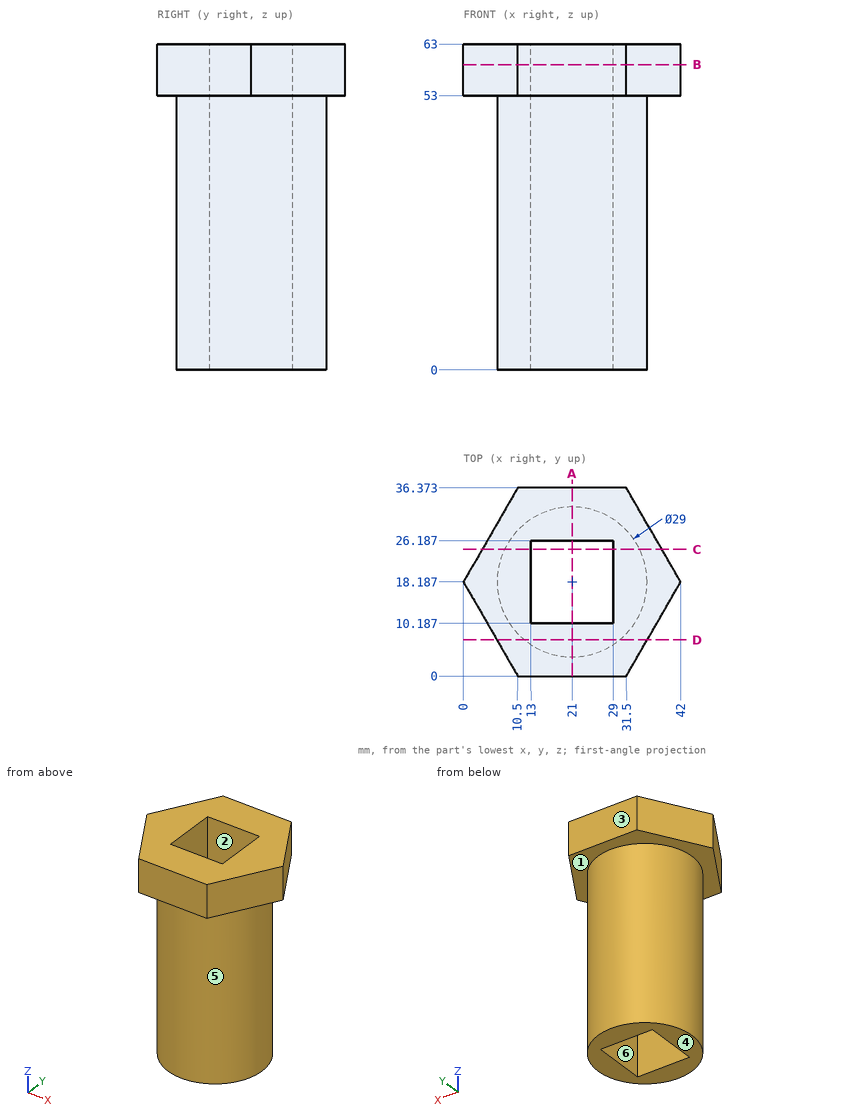
Job drawing, mm, ordinate dimensions from the low corner. One solid piece. A direction names the side the tool comes from. Give positions to 0.01 mm unless a question says otherwise; leave off trailing zeros. Write each loop counter-clockwise with the first axis right and the second up, starting at its lowest first coordinate (ties: lowest second). Pieces come first, ordered by that corner, then holes. Notation, with made-up numbers: (83, 42) - (137, 42) arc R35 cw to (137, 78) - close; hole circle Ø8 at (77, -11). An arc over 180 degrees is marked (long way). Use one line per item in the form item = value. Start each with the question number.
1. Probe line 1 (Z direction, x = 27, y = 2); line 2 (X direction, y = 15, z = 8) (1 decimal); line 3 (Y direction, x = 28, z = 4) (1 decimal). List the from-to ranges inside material, lowest first. Write a range as [from, to].
2. Band-saw the part on A-A on x = 21. Write the cut outline in (y, z).
3. Drop flat-ended pins along their axis: pin 1 Ø1 at (x, z) = (28, 13.5) entering from +Y; pin 2 Ø13 at (x, z) = (25, 35) entering from +Y; pin 3 Ø12 at (y, z) = (20.5, 13.5) entering from +X. Give the stop position or say it passes through.
4. Two-plate mould, pull along X, no slides. Class the marked faces 4, 5 and 6: released by +X, released by -X, zero draft, split by the parting line, or undercut.
5. Band-saw the part on B-B on z = 59. Write the cut outline in (x, y).
6. 3-axis set-ups, long thin cutter, end or side, ignore diameter. For the marked faces 1, 2 and 3: which of +Z, -Z, +X, -X, +Y, -Y reach the whole face in a straight line?
7. Band-saw the part on C-C on y = 24.5. Write the cut outline in (x, z) (1 decimal).
8. Band-saw the part on D-D on y = 7. Write the cut outline in (x, z) (1 decimal), plus the area to 3 significant figures.
Conclusion:
q1.line_1 = [53, 63]
q1.line_2 = [6.9, 13], [29, 35.1]
q1.line_3 = [5.5, 10.2], [26.2, 30.9]
q2.outline = (0, 53) - (3.69, 53) - (3.69, 0) - (10.19, 0) - (10.19, 63) - (0, 63) - close; (26.19, 0) - (32.69, 0) - (32.69, 53) - (36.37, 53) - (36.37, 63) - (26.19, 63) - close
q3.pin_1 = 31.15
q3.pin_2 = 32.69
q3.pin_3 = 35.5
q4.face_4 = zero draft
q4.face_5 = split by the parting line
q4.face_6 = undercut
q5.outline = (0, 18.19) - (10.5, 0) - (31.5, 0) - (42, 18.19) - (31.5, 36.37) - (10.5, 36.37) - close; hole (13, 10.19) - (29, 10.19) - (29, 26.19) - (13, 26.19) - close
q6.face_1 = -Z
q6.face_2 = +Z, -Z
q6.face_3 = +Z, -Z, +X, -X, +Y
q7.outline = (3.6, 53) - (7.9, 53) - (7.9, 0) - (13, 0) - (13, 63) - (3.6, 63) - close; (29, 0) - (34.1, 0) - (34.1, 53) - (38.4, 53) - (38.4, 63) - (29, 63) - close
q8.outline = (6.5, 53) - (11.8, 53) - (11.8, 0) - (30.2, 0) - (30.2, 53) - (35.5, 53) - (35.5, 63) - (6.5, 63) - close
q8.area = 1,270 mm²
